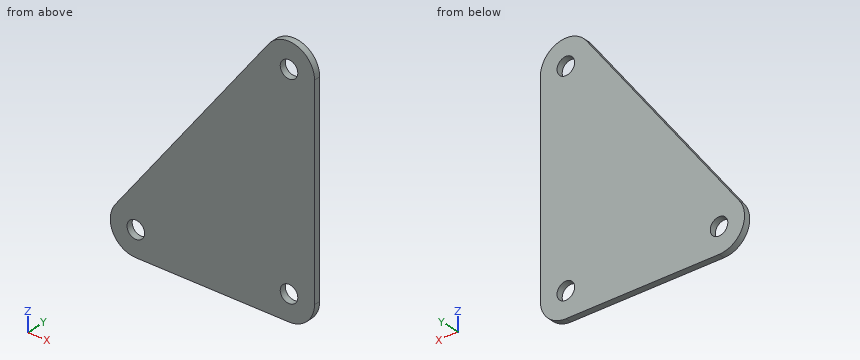
Autodesk Inventor part; units mm, degrees
ref_plane "YZ Plane" through (0, 0, 0) normal (1, 0, 0) x (0, 1, 0)
ref_plane "XZ Plane" through (0, 0, 0) normal (0, 1, 0) x (-1, 0, 0)
ref_plane "XY Plane" through (0, 0, 0) normal (0, 0, 1) x (1, 0, 0)
sketch "main" plane through (0, 0, 0) normal (0, 0, 1) x (1, 0, 0)
  circle A0 centre (-17.594, -20.0255) radius 2.1844
  circle A1 centre (20.506, -20.0255) radius 2.1844
  circle A2 centre (-17.594, 30.7745) radius 2.1844
  arc A3 (-23.944, -20.0255) -> (-17.594, -26.3755) centre (-17.594, -20.0255) ccw
  arc A4 (20.506, -26.3755) -> (25.586, -16.2155) centre (20.506, -20.0255) ccw
  arc A5 (-12.514, 34.5845) -> (-23.944, 30.7745) centre (-17.594, 30.7745) ccw
  line L0 (-17.594, -26.3755) -> (20.506, -26.3755)
  line L1 (-23.944, -20.0255) -> (-23.944, 30.7745)
  line L2 (25.586, -16.2155) -> (-12.514, 34.5845)
  point P0 (-7.053, -5.2935)
  dimension "d0" = 12.7
  dimension "d1" = 12.7
  dimension "d2" = 12.7
sketch "Sketch1" plane through (0, 0, 0) normal (0, 1, 0) x (-1, 0, 0)
  circle A0 centre (0, 0) radius 2.1844
  circle A1 centre (38.1, 0) radius 2.1844
  circle A2 centre (0, 50.8) radius 2.1844
  arc A3 (-6.35, 0) -> (0, -6.35) centre (0, 0) ccw
  arc A4 (38.1, -6.35) -> (43.18, 3.81) centre (38.1, 0) ccw
  arc A5 (5.08, 54.61) -> (-6.35, 50.8) centre (0, 50.8) ccw
  line L0 (0, -6.35) -> (38.1, -6.35)
  line L1 (-6.35, 0) -> (-6.35, 50.8)
  line L2 (43.18, 3.81) -> (5.08, 54.61)
extrude "Extrusion1" add sketch "Sketch1" along normal blind 1.5875
equation "\"BendRadius\" = Thickness"
equation "\"BendReliefWidth\" = Thickness"
equation "\"BendReliefDepth\" = 0.5 * Thickness"
equation "\"CornerReliefSize\" = 4 * Thickness"
equation "\"MinimumRemnant\" = 2 * Thickness"
equation "\"TransitionRadius\" = BendRadius"
equation "\"JacobiRadiusSize\" = BendRadius"
equation "\"GapSize\" = Thickness"
properties part number "intake_gusset" material "Acetal Resin, White"
Geometry check sheet. Reference: the model listing, model coordinates, mm. Give positions to 0.01 mm unless a question says otherwise; leave off trailing zeros. Order: outer loops, then holes, each group sorted by start corner. A loop starts at its lowest first (then second) coordinate and runs counter-clockwise, first axis right, second up. Notation, with made-up numbers: (78.25, -30.75) - (104.25, -30.75) arc R19 cw to (104.25, -22.75) - close; hole circle Ø4 at (72.25, -17). An arc over 180 degrees is marked (long way). Answer as a JSON object with one key per item and string values.
(1) Cross-section at A-A (y = 0.6). Record the cut outline in (x, z), then the cut area to 3 significant figures.
Report:
{"outline": "(-43.18, 3.81) arc R6.35 ccw to (-38.1, -6.35) - (0, -6.35) arc R6.35 ccw to (6.35, 0) - (6.35, 50.8) arc R6.35 ccw to (-5.08, 54.61) - close; hole circle Ø4.37 at (-38.1, 0); hole circle Ø4.37 at (0, 0); hole circle Ø4.37 at (0, 50.8)", "area": "2,020 mm^2"}
(2) Material ranges on line 1 (Z direction, x = 0, y = 0.5); line 2 (Z direction, x = -0.5, y = 0.35); line 3 (Z direction, x = -38.1, y = 0.6), recorded low to high.
Report:
{"line 1": "-6.35 to -2.18, 2.18 to 48.62, 52.98 to 57.15", "line 2": "-6.35 to -2.13, 2.13 to 48.67, 52.93 to 57.13", "line 3": "-6.35 to -2.18, 2.18 to 10.58"}
(3) Cross-section at B-B (x = -10). Record the cut outline in (y, z), then the cut area to 3 significant figures.
Report:
{"outline": "(0, -6.35) - (1.59, -6.35) - (1.59, 48.05) - (0, 48.05) - close", "area": "86.4 mm^2"}
(4) Cross-section at C-C (z = 12). Record the cut outline in (x, y).
Report:
{"outline": "(-37.04, 0) - (6.35, 0) - (6.35, 1.59) - (-37.04, 1.59) - close"}
